Build history of the part. All positions in model axes, mm. A direction names the side the tool comes from. Give positions to 0.01 mm unless a question says otherwise; leave off trailing zeros. Loops run counter-clockwise (first coordinate to the right, second up) from the corner with the lowest first, then second, coordinate; pieces in that order, holes last. Notation, with made-up numbers: M 19.5,37.5 L 39.5,37.5 A24 cw 39.5,60.5 Z; hole C -25,81 d4. An arc over 180 degrees is marked long. Answer as a JSON object with one key per item and string values. Group by question number.
1. Mould opens along X. For faces 3 (the face through (-2.17, -9.76, 12.32)), 4 (the face through (-5, -2, 25)), 5 (the face through (-1.08, -4.88, 20.07)) say: released by +X, released by -X, zero draft, split by the parting line, or undercut.
2. Slice it at A-A (x = 0). List the corners of the cut face in (y, z).
3. Drill centre lines: line 1 along Y through (x, z) = (0, 10); line 2 along Y through (x, z) = (0, 21.75); line 3 along X through (y, z) = (4, 18.75). Where is each one in solid material? Low to high. Write a range as [from, to].
4. Slice it at D-D (x = 4.5). List the corners of the cut face in (y, z), then the cut area to 3 significant figures.
5. 3-axis set-ups, long thin cutter, end or side, ignore diameter. For faces 1 (the face through (2.2, -2.2, 15)), 2 (the face through (2.1, -2.1, 0)): which of +Z, -Z, +X, -X, +Y, -Y reach the whole face in a straight line?
6. Slice it at C-C (z = 19.25). List the corners of the cut face in (x, y), then the cut area to 3 significant figures.
7. Drop flat-ended pins along their axis: pin 1 Ø1 at (x, z) = (-6, 3.5) entering from -Y; pin 2 Ø10 at (y, z) = (7, 6) entering from -X; pin 3 Ø12 at (y, z) = (-7, 6.5) entering from -X. Give the stop position or say it passes through.
from build123d import *

# Parameters (mm, degrees)
SKETCH_R        = 10
PAD_DEPTH       = 25
SKETCH001_R     = 2.75
POCKET_DEPTH    = 25.001
SKETCH002_R     = 5
POCKET001_DEPTH = 10


with BuildPart() as part:
    # Sketch → Pad (new body)
    with BuildSketch(Plane.XY):
        Circle(SKETCH_R)
    extrude(amount=PAD_DEPTH)

    # Sketch001 (on Face3 of Pad) → Pocket (cut, through all)
    with BuildSketch(Plane.XY.offset(25)):
        Circle(SKETCH001_R)
    extrude(amount=-POCKET_DEPTH, mode=Mode.SUBTRACT)

    # Sketch002 (on Face3 of Pocket) → Pocket001 (cut)
    with BuildSketch(Plane.XY.offset(25)):
        Circle(SKETCH002_R)
    extrude(amount=-POCKET001_DEPTH, mode=Mode.SUBTRACT)


solid = part.part
Established:
{
 "1": {"face 3": "split by the parting line", "face 4": "zero draft", "face 5": "undercut"},
 "2": {"outline": "M -10,0 L -2.75,0 L -2.75,15 L -5,15 L -5,25 L -10,25 Z; M 2.75,0 L 10,0 L 10,25 L 5,25 L 5,15 L 2.75,15 Z"},
 "3": {"line 1": "y = [-10, -2.75], [2.75, 10]", "line 2": "y = [-10, -5], [5, 10]", "line 3": "x = [-9.17, -3], [3, 9.17]"},
 "4": {"outline": "M -8.93,0 L 8.93,0 L 8.93,25 L 2.18,25 L 2.18,15 L -2.18,15 L -2.18,25 L -8.93,25 Z", "area": "403 mm^2"},
 "5": {"face 1": "+Z", "face 2": "-Z, +X, -X, +Y, -Y"},
 "6": {"outline": "C 0,0 d20; hole C 0,0 d10", "area": "236 mm^2"},
 "7": {"pin 1": "stops at y = -8.35", "pin 2": "stops at x = -9.8", "pin 3": "stops at x = -9.95"}
}
